The listing builds one solid part. Answer for the finished solid, in the listing's coordinates (mm). A direction names the side the tool comes from. Give positions to 0.01 mm unless a question says otherwise; leave off trailing zeros. Write each loop counter-clockwise with the first axis right and the second up, starting at its lowest first coordinate (ties: lowest second). Pieces come first, ordered by that corner, then holes. Notation, with made-up numbers: (58, 87.5) - (94, 87.5) arc R20 ccw to (94, 102.5) - close; hole circle Ø8 at (37, 56). An arc over 180 degrees is marked (long way). One line per question, with ' | ' between items. Start each with the question number.
1. A cutting plane is placed at B-B (z = -67). Determine the outline of the cut face in (x, y).
2. Find the intervals of material crossed by L1, parallel to Y at x = 0, z = 47; L2, parallel to Z at x = 33, y = -9; L3, parallel to X at y = 5, z = -22.5, in increasing order. Write a range as from..to.
3. A cutting plane is placed at A-A (y = 0). Determine the outline of the cut face in (x, z).
4. The mould has two halves that part along Y. Classify faces 1 (the face through (0, 0, -152.4)), 2 (the face through (3.089, -17.177, 50.889)), 3 (the face through (4.923, -9.464, -75.133)): +Y half, -Y half, draft (parallel to the pull), parting line (faces both ways), or undercut.
5. A cutting plane is placed at C-C (x = 33). Determine the outline of the cut face in (y, z), then the cut area to 3 significant figures.
6. Given P1, Ø3, axis at x = -23, y = 17, coming from the +Z side; P2, Ø3, axis at x = 23.5, z = 9.5, coming from the +Y side; P3, Ø2, axis at x = 0.5, y = -9.5, coming from the +Z side; P4, Ø4.5, axis at x = 0, y = -9.144, coming from the +Z side, each flat-ended and moving along its own axis, determine where each tip first touches the part or whether it passes through.
7. For faces 4 (the face through (0.92, -10.9, 50.89)), 5 (the face through (8, -8, 0)), 6 (the face through (-5.158, -39.287, 6.261)), determine the directions among +Z, -Z, +X, -X, +Y, -Y from which every point of the face is accessible in a straight line to the end or side of a thin tool.
8. A cutting plane is placed at D-D (x = -29.5). Determine the outline of the cut face in (y, z), then the cut area to 3 significant figures.
Autodesk Inventor part; units mm, degrees
ref_plane "Work Plane2" through (0, -13.208, 12.7) normal (-1, 0, 0) x (0, 0, 1)
ref_plane "YZ Plane" through (0, 0, 0) normal (1, 0, 0) x (0, 1, 0)
ref_plane "XZ Plane" through (0, 0, 0) normal (0, 1, 0) x (-1, 0, 0)
sketch "Sketch1" plane through (0, 0, 0) normal (0, 0, 1) x (1, 0, 0)
  circle A0 centre (0, 0) radius 10.668
  dimension "d0" = 21.336
extrude "Extrusion1" add sketch "Sketch1" against normal blind 152.4
sketch "Sketch2" plane through (0, 0, 0) normal (0, 0, 1) x (1, 0, 0)
  circle A0 centre (0, 0) radius 39.624
  dimension "d3" = 79.248
extrude "Extrusion2" add sketch "Sketch2" along normal blind 12.7
sketch "Sketch3" plane through (0, 0, 12.7) normal (0, 0, 1) x (1, 0, 0)
  circle A0 centre (0, -13.208) radius 8.128
  line L0 (0, 0) -> (0, -13.208)
  dimension "d6" = 16.256
  dimension "d7" = 13.208
extrude "Extrusion3" add sketch "Sketch3" along normal blind 44.45
sketch "Sketch10" plane through (0, -13.208, 57.15) normal (0, 0, 1) x (1, 0, 0)
  circle A0 centre (0, 0) radius 6.5405
  point P0 (0, 13.208)
  dimension "d27" = 13.081
extrude "Extrusion6" [suppressed]
sketch "Sketch11" plane through (0, -13.208, 57.15) normal (0, 0, 1) x (1, 0, 0)
  circle A0 centre (0, 0) radius 6.5405
  circle A1 centre (0, 0) radius 8.128
  point P0 (0, 13.208)
  dimension "d30" = 13.081
  dimension "d31" = 16.256
ref_plane "Work Plane2" through (0, -13.208, 12.7) normal (-1, 0, 0) x (0, 0, 1)
sketch "Sketch12" plane through (0, -13.208, 12.7) normal (-1, 0, 0) x (0, 0, 1)
  line L0 (44.45, -8.128) -> (44.45, 8.128)
  line L1 (44.45, 0) -> (57.15, 0)
  line L2 (57.15, 0) -> (69.85, 0) construction
  line L3 (69.85, 0) -> (69.85, 13.208) construction
  line L4 (69.85, 13.208) -> (82.55, 13.208) construction
  spline S0 degree 3 poles (57.15, 0) (69.85, 0) (69.85, 13.208) (82.55, 13.208) knots 1 1 1 1 2 2 2 2
  point P0 (-12.7, 13.208)
  dimension "d32" = 12.7
  dimension "d35" = 13.208
  dimension "d36" = 13.208
  dimension "d37" = 25.4
  dimension "d38" = 12.7
  dimension "d39" = 12.7
sweep "Sweep1" [suppressed]
sketch "Sketch13" plane through (0, 0, 0) normal (0, 1, 0) x (-1, 0, 0)
  line L0 (0, 0) -> (0, 57.15)
  line L1 (8.128, 57.15) -> (-8.128, 57.15)
  circle A0 centre (0, 50.8) radius 1.5875
  circle A1 centre (0, 44.45) radius 1.5875
  circle A2 centre (0, 38.1) radius 1.5875
  circle A3 centre (0, 31.75) radius 1.5875
  circle A4 centre (0, 25.4) radius 1.5875
  point P0 (0, 19.05)
  dimension "d42" = 38.1
  dimension "d43" = 3.175
  dimension "d44" = 6.35
  dimension "d45" = 3.175
  dimension "d46" = 3.175
  dimension "d47" = 3.175
  dimension "d48" = 6.35
  dimension "d49" = 6.35
  dimension "d50" = 6.35
  dimension "d51" = 3.175
  dimension "d52" = 6.35
extrude "Extrusion7" [suppressed]
pattern_circular "Circular Pattern1" [suppressed]
sketch "Sketch14" plane through (0, 0, 0) normal (1, 0, 0) x (0, 1, 0)
  line L0 (0, 0) -> (0, 101.6)
  circle A0 centre (0, 95.25) radius 1.5875
  circle A1 centre (0, 88.9) radius 1.5875
  circle A2 centre (0, 82.55) radius 1.5875
  circle A3 centre (0, 76.2) radius 1.5875
  circle A4 centre (0, 69.85) radius 1.5875
  line L1 (-19.7485, 101.6) -> (-6.6675, 101.6)
  line L2 (-13.208, 101.6) -> (-13.208, 0)
  circle A5 centre (-13.208, 92.075) radius 1.5875
  circle A6 centre (-13.208, 85.725) radius 1.5875
  circle A7 centre (-13.208, 79.375) radius 1.5875
  circle A8 centre (-13.208, 73.025) radius 1.5875
  point P0 (0, 63.5)
  dimension "d59" = 3.175
  dimension "d61" = 3.175
  dimension "d62" = 3.175
  dimension "d63" = 3.175
  dimension "d64" = 6.35
  dimension "d65" = 6.35
  dimension "d66" = 6.35
  dimension "d67" = 3.175
  dimension "d68" = 6.35
  dimension "d69" = 3.175
  dimension "d70" = 3.175
  dimension "d71" = 3.175
  dimension "d72" = 3.175
  dimension "d73" = 9.525
  dimension "d74" = 6.35
  dimension "d75" = 6.35
  dimension "d76" = 6.35
extrude "Extrusion8" [suppressed]
pattern_circular "Circular Pattern2" [suppressed]
sketch "Sketch15" plane through (0, -13.208, 57.15) normal (0, 0, 1) x (1, 0, 0)
  circle A0 centre (0, 4.064) radius 1.9844
  line L0 (0, 4.064) -> (0, 13.208)
  dimension "d82" = 9.144
  dimension "d83" = 3.9688
extrude "Extrusion9" cut sketch "Sketch15" against normal blind 12.7
pattern_circular "Circular Pattern3" count 3 over 360 about axis through (0, -13.208, 12.7) along (0, 0, 1) of "Extrusion9"
equation "\"d1\" = 3.81 * scale"
equation "\"d3\" = 1.9812 * scale"
equation "\"d4\" = 0.3175 * scale"
equation "\"d6\" = 0.4064 * scale"
equation "\"d7\" = 0.3302 * scale"
equation "\"d8\" = 1.11125 * scale"
equation "\"d35\" = 0.3302 * scale"
equation "\"d36\" = 0.3302 * scale"
equation "\"d53\" = 0.3302 * scale"
equation "\"d77\" = 0.3302 * scale"
equation "\"d82\" = 0.2286 * scale"
equation "\"d84\" = 0.3175 * scale"
equation "\"radius\" = 3.175"
properties part number "Eccentric_Shaft_2" material "Stainless Steel"
Determined:
1) outline: circle Ø21.34 at (0, 0)
2) L1: -21.34..-11.13, -7.16..-5.08 | L2: 0..12.7 | L3: -9.42..9.42
3) outline: (-39.62, 0) - (-10.67, 0) - (-10.67, -152.4) - (10.67, -152.4) - (10.67, 0) - (39.62, 0) - (39.62, 12.7) - (-39.62, 12.7) - close
4) face 1: draft | face 2: undercut | face 3: parting line
5) outline: (-21.93, 0) - (21.93, 0) - (21.93, 12.7) - (-21.93, 12.7) - close | area: 557 mm2
6) P1: z = 12.7 | P2: y = 32.96 | P3: z = 44.45 | P4: z = 57.15
7) face 4: +Z | face 5: -Z | face 6: +Z, -Z
8) outline: (-26.45, 0) - (26.45, 0) - (26.45, 12.7) - (-26.45, 12.7) - close | area: 672 mm2
